Model file for the job. Use its own axes, mm. Face numbers are marked on the shaded views. A direction names the side the tool comes from. Give positions to 0.01 mm unless a question says otherwise; leave off trailing zeros. Write each loop counter-clockwise with the first axis right and the second up, starting at its lowest first coordinate (ties: lowest second). Pieces come first, ordered by that corner, then holes. Notation, with made-up numbers: (64.25, 39.5) - (92.25, 39.5) arc R35 ccw to (92.25, 73.5) - close; hole circle Ø4 at (31, 36). An arc over 180 degrees is marked (long way). One line per item, written item: value. Start each with the question number.
(1) Drop flat-ended pins along their axis: P1, Ø12.5, axis at x = -23.5, z = 12, coming from the -Y side; P2, Ø12.5, axis at x = -96.5, z = 10, coming from the +Y side; P3, Ø2, axis at y = -123.5, z = 4, coming from the +X side. Give the stop position or say it passes through.
(2) Cut at A-A, the plane x = 0. List the corners of the cut face in (y, z).
(3) Mould opens along Y. For the marked faces 1, 2, 3 and 4 say: pulls with the +Y half, pulls with the -Y half, needs draft (parallel to the pull), parting line crosses it, or undercut.
(4) Cut at D-D, the plane x = -119. List the corners of the cut face in (y, z).
(5) Cut at C-C, the plane y = 39. List the corners of the cut face in (x, z), and give its area (3 significant figures).
(6) Cut at B-B, the plane z = 5.5. State how many separate pieces and enclosed holes the cut face has, and give its area (3 significant figures).
(7) 3-axis set-ups, long thin cutter, end or side, ignore diameter. For the marked faces 5, 6 and 7: which of +Z, -Z, +X, -X, +Y, -Y reach the whole face in a straight line?
(8) Probe L1, parallel to X at y = -6.5, z = 13.25; L2, parallel to Y at x = -70, z = 18.5; L3, parallel to Y at x = -64, z = 24.25. List the from-to ranges inside material, lowest first.
from build123d import *

# Parameters (mm, degrees)
F0_R     = 15
F0_R_2   = 1.6
F0_W     = 102
F0_H     = 29.597664
F1_DEPTH = 25
F2_DEPTH = 25


with BuildPart() as f1:
    # F0 (on Top) → F1 (new body)
    with BuildSketch(Plane.XY):
        with BuildLine():
            Line((76, 93.350048), (0, 93.350048))
            Line((0, 93.350048), (-76, 93.350048))
            Line((-76, 93.350048), (-76, 28.350048))
            Line((-76, 28.350048), (-136, 28.350048))
            Line((-136, 28.350048), (-136, -76.986715))
            ThreePointArc((-136, -76.986715), (-133.398174, -86.850972), (-126.269644, -94.14872))
            ThreePointArc((-126.269644, -94.14872), (0, -181.145858), (126.269644, -94.14872))
            ThreePointArc((126.269644, -94.14872), (133.398174, -86.850972), (136, -76.986715))
            Line((136, -76.986715), (136, 28.350048))
            Line((136, 28.350048), (76, 28.350048))
            Line((76, 28.350048), (76, 93.350048))
        make_face()
        with Locations((0, -46.011958)):
            Circle(F0_R, mode=Mode.SUBTRACT)
        with Locations((-59.481014, 5.299877)):
            Circle(F0_R_2, mode=Mode.SUBTRACT)
        with Locations((-0.031014, 5.299877)):
            Rectangle(F0_W, F0_H, mode=Mode.SUBTRACT)
        with Locations((-70, 58.350048)):
            Circle(F0_R_2, mode=Mode.SUBTRACT)
        with Locations((-70, 87.350048)):
            Circle(F0_R_2, mode=Mode.SUBTRACT)
        with Locations((-64, 58.350048)):
            Circle(F0_R_2, mode=Mode.SUBTRACT)
        with Locations((-58, 58.350048)):
            Circle(F0_R_2, mode=Mode.SUBTRACT)
        with Locations((-64, 87.350048)):
            Circle(F0_R_2, mode=Mode.SUBTRACT)
        with Locations((-58, 87.350048)):
            Circle(F0_R_2, mode=Mode.SUBTRACT)
        with Locations((59.418986, 5.299877)):
            Circle(F0_R_2, mode=Mode.SUBTRACT)
        with Locations((56.15901, 58.350048)):
            Circle(F0_R_2, mode=Mode.SUBTRACT)
        with Locations((62.15901, 58.350048)):
            Circle(F0_R_2, mode=Mode.SUBTRACT)
        with Locations((56.15901, 87.350048)):
            Circle(F0_R_2, mode=Mode.SUBTRACT)
        with Locations((62.15901, 87.350048)):
            Circle(F0_R_2, mode=Mode.SUBTRACT)
        with Locations((68.15901, 58.350048)):
            Circle(F0_R_2, mode=Mode.SUBTRACT)
        with Locations((68.15901, 87.350048)):
            Circle(F0_R_2, mode=Mode.SUBTRACT)
    extrude(amount=F1_DEPTH)

    # F0 (on Top) → F2 (join)
    with BuildSketch(Plane.XY):
        with BuildLine():
            Line((76, 93.350048), (0, 93.350048))
            Line((0, 93.350048), (-76, 93.350048))
            Line((-76, 93.350048), (-76, 28.350048))
            Line((-76, 28.350048), (-136, 28.350048))
            Line((-136, 28.350048), (-136, -76.986715))
            ThreePointArc((-136, -76.986715), (-133.398174, -86.850972), (-126.269644, -94.14872))
            ThreePointArc((-126.269644, -94.14872), (0, -181.145858), (126.269644, -94.14872))
            ThreePointArc((126.269644, -94.14872), (133.398174, -86.850972), (136, -76.986715))
            Line((136, -76.986715), (136, 28.350048))
            Line((136, 28.350048), (76, 28.350048))
            Line((76, 28.350048), (76, 93.350048))
        make_face()
        with Locations((0, -46.011958)):
            Circle(F0_R, mode=Mode.SUBTRACT)
        with Locations((-59.481014, 5.299877)):
            Circle(F0_R_2, mode=Mode.SUBTRACT)
        with Locations((-0.031014, 5.299877)):
            Rectangle(F0_W, F0_H, mode=Mode.SUBTRACT)
        with Locations((-70, 58.350048)):
            Circle(F0_R_2, mode=Mode.SUBTRACT)
        with Locations((-70, 87.350048)):
            Circle(F0_R_2, mode=Mode.SUBTRACT)
        with Locations((-64, 58.350048)):
            Circle(F0_R_2, mode=Mode.SUBTRACT)
        with Locations((-58, 58.350048)):
            Circle(F0_R_2, mode=Mode.SUBTRACT)
        with Locations((-64, 87.350048)):
            Circle(F0_R_2, mode=Mode.SUBTRACT)
        with Locations((-58, 87.350048)):
            Circle(F0_R_2, mode=Mode.SUBTRACT)
        with Locations((59.418986, 5.299877)):
            Circle(F0_R_2, mode=Mode.SUBTRACT)
        with Locations((56.15901, 58.350048)):
            Circle(F0_R_2, mode=Mode.SUBTRACT)
        with Locations((62.15901, 58.350048)):
            Circle(F0_R_2, mode=Mode.SUBTRACT)
        with Locations((56.15901, 87.350048)):
            Circle(F0_R_2, mode=Mode.SUBTRACT)
        with Locations((62.15901, 87.350048)):
            Circle(F0_R_2, mode=Mode.SUBTRACT)
        with Locations((68.15901, 58.350048)):
            Circle(F0_R_2, mode=Mode.SUBTRACT)
        with Locations((68.15901, 87.350048)):
            Circle(F0_R_2, mode=Mode.SUBTRACT)
    extrude(amount=F2_DEPTH)


solid = f1.part
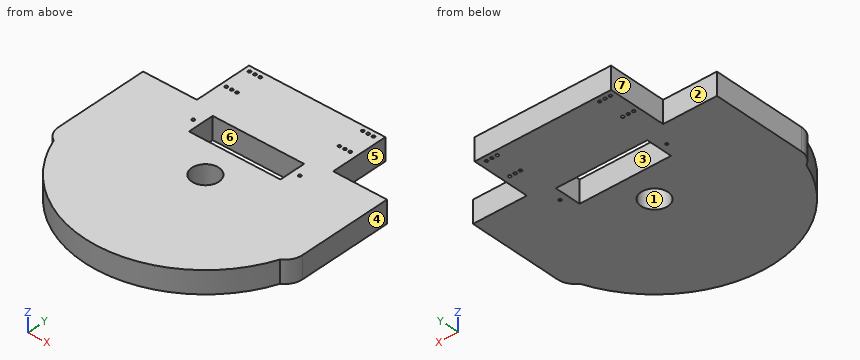
Answers follow:
1. P1: stops at y = -180.04
1. P2: stops at y = 28.35
1. P3: stops at x = 111.4
2. outline: (-181.15, 0) - (-61.01, 0) - (-61.01, 25) - (-181.15, 25) - close; (-31.01, 0) - (-9.5, 0) - (-9.5, 25) - (-31.01, 25) - close; (20.1, 0) - (93.35, 0) - (93.35, 25) - (20.1, 25) - close
3. face 1: undercut
3. face 2: pulls with the +Y half
3. face 3: undercut
3. face 4: needs draft
4. outline: (-110.04, 0) - (28.35, 0) - (28.35, 25) - (-110.04, 25) - close
5. outline: (-76, 0) - (76, 0) - (76, 25) - (-76, 25) - close
5. area: 3,800 mm²
6. separate pieces: 1
6. enclosed holes: 16
6. area: 55,200 mm²
7. face 5: +Z, -Z, +X, +Y
7. face 6: +Z, -Z
7. face 7: +Z, -Z, -X, +Y
8. L1: x = -136 to -51.03, 50.97 to 136
8. L2: y = -161.6 to 56.75, 59.95 to 85.75, 88.95 to 93.35
8. L3: y = -165.03 to 56.75, 59.95 to 85.75, 88.95 to 93.35
